```python
from build123d import *

# Parameters (mm, degrees)
SKETCH1_W           = 12.5
SKETCH1_H           = 23
BOSS_EXTRUDE1_DEPTH = 5
SKETCH4_W           = 3.25
SKETCH4_H           = 1.4
CUT_EXTRUDE1_DEPTH  = 44.732139211


# Read off the part's stored shape, not the designer's step: CSK for M2 Flat Head Machine Screw1
with BuildPart() as part:
    # Sketch1 → Boss-Extrude1 (new, symmetric)
    with BuildSketch(Plane(origin=(0, 0, 0), x_dir=(0, 0, -1), z_dir=(1, 0, 0))):
        Polygon((-9.5, -16.5), (-3.266799929, -41.5), (6.508063966, -41.5), (6.508063966, -28.5), (9.5, -16.5), (9.5, 16.5), (-9.5, 16.5), align=None)
        Rectangle(SKETCH1_W, SKETCH1_H, mode=Mode.SUBTRACT)
    extrude(amount=BOSS_EXTRUDE1_DEPTH, both=True)

    # CSK for M2 Flat Head Machine Screw1 outl → CSK for M2 Flat Head Machine Screw1 (revolve, cut)
    with BuildSketch(Plane(origin=(0, 13.9, 0), x_dir=(0, 1, 0), z_dir=(0, 0, -1))):
        Polygon((0.87, 3), (0, 3.522748739), (0, -5), (1.5, -5), (0.87, -4.37), align=None)
    revolve(axis=Axis((0, 13.9, 0), (1, 0, 0)), mode=Mode.SUBTRACT)

    # CSK for M2 Flat Head Machine Screw1 2 ou → CSK for M2 Flat Head Machine Screw1 2 (revolve, cut)
    with BuildSketch(Plane(origin=(0, -13.9, 0), x_dir=(0, 1, 0), z_dir=(0, 0, -1))):
        Polygon((0.87, 3), (0, 3.522748739), (0, -5), (1.5, -5), (0.87, -4.37), align=None)
    revolve(axis=Axis((0, -13.9, 0), (1, 0, 0)), mode=Mode.SUBTRACT)

    # Sketch4 → Cut-Extrude1 (cut, through all)
    with BuildSketch(Plane(origin=(5, 0, 0), x_dir=(0, 0, -1), z_dir=(1, 0, 0))):
        with Locations((-7.875, 10.8)):
            Rectangle(SKETCH4_W, SKETCH4_H)
    extrude(amount=-CUT_EXTRUDE1_DEPTH, mode=Mode.SUBTRACT)


solid = part.part
```
Geometry: final body of the model. Coordinates: model frame, mm. A direction names the side the tool comes from. Round coordinates to 2 decimals unless told otherwise and drop trailing zeros. Loops run counter-clockwise (first coordinate to the right, second up) from the corner with the lowest first, then second, coordinate; pieces in that order, holes last. Notation, with made-up numbers: (26.25, 0.5) -> (48.25, 0.5) arc R28 ccw to (48.25, 18.5) -> close; hole circle Ø2 at (81, -8). An arc over 180 degrees is marked (long way). Write each question's results on one line, items separated by ' | '.
Item 1: Set-up query: faces 5 (the face through (-0.63, 14.73, 0.26)), 6 (the face through (0, -35, -6.508)), 7 (the face through (0, 10.1, 8)), 8 (the face through (5, -12, 0)), 9 (the face through (0, 0, -6.25)). Return all of +Z, -Z, +X, -X, +Y, -Y with unobstructed straight access to the full face (end or side cutting, diameter ignored); none if empty.
Answers below:
face 5: -X | face 6: -Z, +X, -X, -Y | face 7: +Z, +X, -X | face 8: +Z, -Z, +X, +Y, -Y | face 9: +X, -X
Item 2: Pull-direction query (Y, two-part tool) for faces 1 (the face through (0, 16.5, 0)), 2 (the face through (-0.63, -14.77, 0.04)), 3 (the face through (0, 0, -9.5)), 4 (the face through (0, 11.5, 2)); classes: pulls with the +Y half, pulls with the -Y half, needs draft (parallel to the pull), parting line crosses it, or undercut.
Answers below:
face 1: pulls with the +Y half | face 2: undercut | face 3: needs draft | face 4: undercut
Item 3: Cut plane C-C on x = 2.5. Return the cut outline in (y, z).
Answers below:
outline: (-41.5, -6.51) -> (-28.5, -6.51) -> (-16.5, -9.5) -> (16.5, -9.5) -> (16.5, 9.5) -> (11.5, 9.5) -> (11.5, -6.25) -> (-11.5, -6.25) -> (-11.5, 6.25) -> (10.1, 6.25) -> (10.1, 9.5) -> (-16.5, 9.5) -> (-41.5, 3.27) -> close; hole circle Ø1.74 at (-13.9, 0); hole circle Ø1.74 at (13.9, 0)
Item 4: Cut plane A-A on z = -4.25. Return the cut outline in (x, y).
Answers below:
outline: (-5, -41.5) -> (5, -41.5) -> (5, -11.5) -> (-5, -11.5) -> close; (-5, 11.5) -> (5, 11.5) -> (5, 16.5) -> (-5, 16.5) -> close
Item 5: Line query: probe 1 along Y at (x, z) = (-4, 3); probe 2 along Z at (x, y) = (-2.5, -8.5); probe 3 along Y at (x, z) = (2.5, -0.5). Output: solid intervals per line, ascending. Write a range as [from, to].
Answers below:
probe 1: y = [-41.5, -11.5], [11.5, 16.5] | probe 2: z = [-9.5, -6.25], [6.25, 9.5] | probe 3: y = [-41.5, -14.61], [-13.19, -11.5], [11.5, 13.19], [14.61, 16.5]
Item 6: Pin query (flat end, axial travel): pin 1 Ø6 at (x, z) = (2, 6) entering from -Y; pin 2 Ø1.4 at (y, z) = (13.9, 0) entering from -X; pin 3 Ø5 at (x, y) = (-2, -33.5) entering from -Z. Return the tip coordinate at first contact, or that it passes through.
Answers below:
pin 1: stops at y = -41.5 | pin 2: stops at x = 3.1 | pin 3: stops at z = -6.51
Item 7: Cut plane B-B on y = -10.5. Return the cut outline in (x, z).
Answers below:
outline: (-5, -9.5) -> (5, -9.5) -> (5, -6.25) -> (-5, -6.25) -> close; (-5, 6.25) -> (5, 6.25) -> (5, 9.5) -> (-5, 9.5) -> close
